```python
from build123d import *

# Parameters (mm, degrees)
SKETCH_1_W          = 200
SKETCH_1_H          = 268
EXTRUDE_1_DEPTH     = 4
CUT_EXTRUDE_1_DEPTH = 5


with BuildPart() as part:
    # 草图1 → 凸台-拉伸1 (new body)
    with BuildSketch(Plane.XY):
        Rectangle(SKETCH_1_W, SKETCH_1_H)
    extrude(amount=EXTRUDE_1_DEPTH)

    # 草图2 → 切除-拉伸1 (cut, through all)
    with BuildSketch(Plane.XY.offset(4)):
        with BuildLine():
            Line((-75, 115.5), (75, 115.5))
            ThreePointArc((75, 115.5), (82.5, 108), (75, 100.5))
            Line((75, 100.5), (-75, 100.5))
            ThreePointArc((-75, 100.5), (-82.5, 108), (-75, 115.5))
        make_face()
        with BuildLine():
            Line((-75, 61.5), (75, 61.5))
            ThreePointArc((75, 61.5), (82.5, 54), (75, 46.5))
            Line((75, 46.5), (-75, 46.5))
            ThreePointArc((-75, 46.5), (-82.5, 54), (-75, 61.5))
        make_face()
        with BuildLine():
            Line((-75, 7.5), (75, 7.5))
            ThreePointArc((75, 7.5), (82.5, 0), (75, -7.5))
            Line((75, -7.5), (-75, -7.5))
            ThreePointArc((-75, -7.5), (-82.5, 0), (-75, 7.5))
        make_face()
        with BuildLine():
            Line((-75, -46.5), (75, -46.5))
            ThreePointArc((75, -46.5), (82.5, -54), (75, -61.5))
            Line((75, -61.5), (-75, -61.5))
            ThreePointArc((-75, -61.5), (-82.5, -54), (-75, -46.5))
        make_face()
        with BuildLine():
            Line((-75, -100.5), (75, -100.5))
            ThreePointArc((75, -100.5), (82.5, -108), (75, -115.5))
            Line((75, -115.5), (-75, -115.5))
            ThreePointArc((-75, -115.5), (-82.5, -108), (-75, -100.5))
        make_face()
    extrude(amount=-CUT_EXTRUDE_1_DEPTH, mode=Mode.SUBTRACT)


solid = part.part
```
Check sheet for the modelled part. Datum: model origin and axes. Units: mm. A direction names the side the tool comes from. Round coordinates to 2 decimals unless told otherwise and drop trailing zeros. Order: outer loops, then holes, each group sorted by start corner. A loop starts at its lowest first (then second) coordinate and runs counter-clockwise, first axis right, second up. Notation, with made-up numbers: (78.5, 14) -> (86.5, 14) arc R20 cw to (86.5, 34) -> close; hole circle Ø5 at (74, 31). An arc over 180 degrees is marked (long way). Use CSV: the item, a comma, the result in double quotes.
(1) Material ranges on line 1 along Y through (x, z) = (46.5, 2.6); line 2 along X through (y, z) = (-114.5, 2.7); line 3 along X through (y, z) = (-105.5, 3.8), recorded low to high. Write a range as from..to.
Worked out:
line 1,"-134..-115.5, -100.5..-61.5, -46.5..-7.5, 7.5..46.5, 61.5..100.5, 115.5..134"
line 2,"-100..-78.74, 78.74..100"
line 3,"-100..-82.07, 82.07..100"
(2) Cross-section at C-C (y = 0). Record the boundary of the cut face in (x, z), and give its area (3 significant figures).
Worked out:
outline,"(-100, 0) -> (-82.5, 0) -> (-82.5, 4) -> (-100, 4) -> close; (82.5, 0) -> (100, 0) -> (100, 4) -> (82.5, 4) -> close"
area,"140 mm²"
(3) Cross-section at B-B (x = 3). Record the boundary of the cut face in (y, z), and give its area (3 significant figures).
Worked out:
outline,"(-134, 0) -> (-115.5, 0) -> (-115.5, 4) -> (-134, 4) -> close; (-100.5, 0) -> (-61.5, 0) -> (-61.5, 4) -> (-100.5, 4) -> close; (-46.5, 0) -> (-7.5, 0) -> (-7.5, 4) -> (-46.5, 4) -> close; (7.5, 0) -> (46.5, 0) -> (46.5, 4) -> (7.5, 4) -> close; (61.5, 0) -> (100.5, 0) -> (100.5, 4) -> (61.5, 4) -> close; (115.5, 0) -> (134, 0) -> (134, 4) -> (115.5, 4) -> close"
area,"772 mm²"
(4) Cross-section at A-A (z = 0.9). Record the boundary of the cut face in (x, y).
Worked out:
outline,"(-100, -134) -> (100, -134) -> (100, 134) -> (-100, 134) -> close; hole (-75, -115.5) -> (75, -115.5) arc R7.5 ccw to (75, -100.5) -> (-75, -100.5) arc R7.5 ccw to start; hole (-75, -61.5) -> (75, -61.5) arc R7.5 ccw to (75, -46.5) -> (-75, -46.5) arc R7.5 ccw to start; hole (-75, -7.5) -> (75, -7.5) arc R7.5 ccw to (75, 7.5) -> (-75, 7.5) arc R7.5 ccw to start; hole (-75, 46.5) -> (75, 46.5) arc R7.5 ccw to (75, 61.5) -> (-75, 61.5) arc R7.5 ccw to start; hole (-75, 100.5) -> (75, 100.5) arc R7.5 ccw to (75, 115.5) -> (-75, 115.5) arc R7.5 ccw to start"
(5) Tool access check on faces 1 (the face through (-82.5, 53.84, 2.03)), 2 (the face through (-1, 32, 4)). Record the directions out of +Z, -Z, +X, -X, +Y, -Y that give a thin tool (end or side, any length) a straight path to the whole face; none if there is none.
Worked out:
face 1,"+Z, -Z"
face 2,"+Z, +X, -X, +Y, -Y"
(6) Draft check along X on faces 3 (the face through (82.5, -107.84, 2.03)), 4 (the face through (-1, 32, 0)). Enter one of: pulls with the +X half, pulls with the -X half, needs draft (parallel to the pull), parting line crosses it, or undercut.
Worked out:
face 3,"undercut"
face 4,"needs draft"
